Input: part model. Units: mm. Frame: model coordinates. A direction names the side the tool comes from. Round coordinates to 2 decimals unless told otherwise and drop trailing zeros. Write each loop counter-clockwise with the first axis right and the second up, starting at its lowest first coordinate (ties: lowest second). Pieces come first, ordered by that corner, then holes. Notation, with made-up numbers: M -37,-7 L -10,-7 A19 ccw -10,2 Z; hole C 53.5,17.25 d1. An arc over 180 degrees is marked long. Use one line per item in the form item = value. Start each with the question number.
```python
from build123d import *

# Parameters (mm, degrees)
F1_DEPTH  = 3.7
F2_DEPTH  = 55.6
F5_DEPTH  = 5
F7_D      = 3.15
F7_DEPTH  = 10
F7_TIP    = 0.946355475
F9_R      = 3
F10_DEPTH = 10
F12_DEPTH = 5
F11_R     = 2.5
F13_DEPTH = 25
F11_R_2   = 3.5
F14_DEPTH = 1
F15_SIZE  = 4
F16_W     = 4.2
F16_H     = 8
F16_W_2   = 6.1
F16_H_2   = 14
F17_DEPTH = 1
F18_DEPTH = 3
F19_R     = 0.8


with BuildPart() as f1:
    # F0 (on Top) → F1 (new body)
    with BuildSketch(Plane.XY):
        with BuildLine():
            ThreePointArc((43.1, 37.5), (39.2923881554, 46.6923881554), (30.1, 50.5))
            Line((30.1, 50.5), (-35.1, 50.5))
            ThreePointArc((-35.1, 50.5), (-40.7568542495, 48.1568542495), (-43.1, 42.5))
            Line((-43.1, 42.5), (-43.1, -37.5))
            ThreePointArc((-43.1, -37.5), (-39.2923881554, -46.6923881554), (-30.1, -50.5))
            Line((-30.1, -50.5), (30.1, -50.5))
            ThreePointArc((30.1, -50.5), (39.2923881554, -46.6923881554), (43.1, -37.5))
            Line((43.1, -37.5), (43.1, 37.5))
        make_face()
        with BuildLine():
            Line((40.1, 37.5), (40.1, 27.7))
            Line((40.1, 27.7), (40.1, -37.5))
            ThreePointArc((40.1, -37.5), (37.1710678119, -44.5710678119), (30.1, -47.5))
            Line((30.1, -47.5), (-30.1, -47.5))
            ThreePointArc((-30.1, -47.5), (-37.1710678119, -44.5710678119), (-40.1, -37.5))
            Line((-40.1, -37.5), (-40.1, 27.7))
            Line((-40.1, 27.7), (-40.1, 42.5))
            ThreePointArc((-40.1, 42.5), (-38.6355339059, 46.0355339059), (-35.1, 47.5))
            Line((-35.1, 47.5), (30.1, 47.5))
            ThreePointArc((30.1, 47.5), (37.1710678119, 44.5710678119), (40.1, 37.5))
        make_face(mode=Mode.SUBTRACT)
        with BuildLine():
            Line((-30.1, 37.7), (30.1, 37.7))
            ThreePointArc((30.1, 37.7), (37.1710678119, 34.7710678119), (40.1, 27.7))
            Line((40.1, 27.7), (40.1, 37.5))
            ThreePointArc((40.1, 37.5), (37.1710678119, 44.5710678119), (30.1, 47.5))
            Line((30.1, 47.5), (-35.1, 47.5))
            ThreePointArc((-35.1, 47.5), (-38.6355339059, 46.0355339059), (-40.1, 42.5))
            Line((-40.1, 42.5), (-40.1, 27.7))
            ThreePointArc((-40.1, 27.7), (-37.1710678119, 34.7710678119), (-30.1, 37.7))
        make_face()
    extrude(amount=F1_DEPTH)

    # F0 (on Top) → F2 (join)
    with BuildSketch(Plane.XY):
        with BuildLine():
            ThreePointArc((43.1, 37.5), (39.2923881554, 46.6923881554), (30.1, 50.5))
            Line((30.1, 50.5), (-35.1, 50.5))
            ThreePointArc((-35.1, 50.5), (-40.7568542495, 48.1568542495), (-43.1, 42.5))
            Line((-43.1, 42.5), (-43.1, -37.5))
            ThreePointArc((-43.1, -37.5), (-39.2923881554, -46.6923881554), (-30.1, -50.5))
            Line((-30.1, -50.5), (30.1, -50.5))
            ThreePointArc((30.1, -50.5), (39.2923881554, -46.6923881554), (43.1, -37.5))
            Line((43.1, -37.5), (43.1, 37.5))
        make_face()
        with BuildLine():
            Line((40.1, 37.5), (40.1, 27.7))
            Line((40.1, 27.7), (40.1, -37.5))
            ThreePointArc((40.1, -37.5), (37.1710678119, -44.5710678119), (30.1, -47.5))
            Line((30.1, -47.5), (-30.1, -47.5))
            ThreePointArc((-30.1, -47.5), (-37.1710678119, -44.5710678119), (-40.1, -37.5))
            Line((-40.1, -37.5), (-40.1, 27.7))
            Line((-40.1, 27.7), (-40.1, 42.5))
            ThreePointArc((-40.1, 42.5), (-38.6355339059, 46.0355339059), (-35.1, 47.5))
            Line((-35.1, 47.5), (30.1, 47.5))
            ThreePointArc((30.1, 47.5), (37.1710678119, 44.5710678119), (40.1, 37.5))
        make_face(mode=Mode.SUBTRACT)
    extrude(amount=F2_DEPTH)

    # F4 (on offset) → F5 (join, symmetric)
    with BuildSketch(Plane(origin=(0, 0, 0), x_dir=(0, -1, 0), z_dir=(-1, 0, 0))):
        Polygon((47.5, 45.6), (47.5, 55.6), (37.5, 55.6), (37.5, 52.6), align=None)
        Polygon((-37.5, 52.6), (-37.5, 55.6), (-47.5, 55.6), (-47.5, 45.6), align=None)
    extrude(amount=F5_DEPTH, both=True)

    # F7
    with Locations(Plane.XY.offset(55.6)):
        with Locations((0, 42.5), (0, -42.5)):
            Hole(F7_D / 2, depth=F7_DEPTH)
            with Locations((0, 0, -(F7_DEPTH + F7_TIP / 2))):  # 118° drill point
                Cone(0, F7_D / 2, F7_TIP, mode=Mode.SUBTRACT)

    # F9 (on offset) → F10 (cut)
    with BuildSketch(Plane.XY.offset(52.6)):
        with Locations((0, 42.5)):
            Circle(F9_R)
        with Locations((0, -42.5)):
            Circle(F9_R)
    extrude(amount=-F10_DEPTH, mode=Mode.SUBTRACT)

    # F11 (on face) → F12 (join)
    with BuildSketch(Plane.XZ.offset(-47.5)):
        with BuildLine():
            ThreePointArc((-29.1, 37.3270166538), (-26.9377223398, 38.7505102572), (-26.1, 41.2))
            ThreePointArc((-26.1, 41.2), (-32.5494897428, 44.3622776602), (-31.1, 37.3270166538))
            ThreePointArc((-31.1, 37.3270166538), (-30.1, 37.2), (-29.1, 37.3270166538))
        make_face()
        Polygon((-30.1, 44.3754264805), (-27.35, 42.7877132403), (-27.35, 39.6122867597), (-30.1, 38.0245735195), (-32.85, 39.6122867597), (-32.85, 42.7877132403), align=None, mode=Mode.SUBTRACT)
        with BuildLine():
            ThreePointArc((-29.1, 37.3270166538), (-30.1, 37.2), (-31.1, 37.3270166538))
            Line((-31.1, 37.3270166538), (-31.1, 33.2))
            Line((-31.1, 33.2), (-29.1, 33.2))
            Line((-29.1, 33.2), (-29.1, 37.3270166538))
        make_face()
        with BuildLine():
            ThreePointArc((2.9, 37.3270166538), (5.0622776602, 38.7505102572), (5.9, 41.2))
            ThreePointArc((5.9, 41.2), (-0.5494897428, 44.3622776602), (0.9, 37.3270166538))
            ThreePointArc((0.9, 37.3270166538), (1.9, 37.2), (2.9, 37.3270166538))
        make_face()
        Polygon((1.9, 44.3754264805), (4.65, 42.7877132403), (4.65, 39.6122867597), (1.9, 38.0245735195), (-0.85, 39.6122867597), (-0.85, 42.7877132403), align=None, mode=Mode.SUBTRACT)
        with BuildLine():
            ThreePointArc((2.9, 37.3270166538), (1.9, 37.2), (0.9, 37.3270166538))
            Line((0.9, 37.3270166538), (0.9, 33.2))
            Line((0.9, 33.2), (2.9, 33.2))
            Line((2.9, 33.2), (2.9, 37.3270166538))
        make_face()
        with BuildLine():
            ThreePointArc((-27.1, 8.3270166538), (-24.9377223398, 9.7505102572), (-24.1, 12.2))
            ThreePointArc((-24.1, 12.2), (-30.5494897428, 15.3622776602), (-29.1, 8.3270166538))
            ThreePointArc((-29.1, 8.3270166538), (-28.1, 8.2), (-27.1, 8.3270166538))
        make_face()
        Polygon((-28.1, 15.3754264805), (-25.35, 13.7877132403), (-25.35, 10.6122867597), (-28.1, 9.0245735195), (-30.85, 10.6122867597), (-30.85, 13.7877132403), align=None, mode=Mode.SUBTRACT)
        with BuildLine():
            ThreePointArc((-27.1, 8.3270166538), (-28.1, 8.2), (-29.1, 8.3270166538))
            Line((-29.1, 8.3270166538), (-29.1, 6.2))
            Line((-29.1, 6.2), (-27.1, 6.2))
            Line((-27.1, 6.2), (-27.1, 8.3270166538))
        make_face()
        with BuildLine():
            ThreePointArc((5.9, 8.3270166538), (8.0622776602, 9.7505102572), (8.9, 12.2))
            ThreePointArc((8.9, 12.2), (2.4505102572, 15.3622776602), (3.9, 8.3270166538))
            ThreePointArc((3.9, 8.3270166538), (4.9, 8.2), (5.9, 8.3270166538))
        make_face()
        Polygon((4.9, 15.3754264805), (7.65, 13.7877132403), (7.65, 10.6122867597), (4.9, 9.0245735195), (2.15, 10.6122867597), (2.15, 13.7877132403), align=None, mode=Mode.SUBTRACT)
        with BuildLine():
            ThreePointArc((5.9, 8.3270166538), (4.9, 8.2), (3.9, 8.3270166538))
            Line((3.9, 8.3270166538), (3.9, 6.2))
            Line((3.9, 6.2), (5.9, 6.2))
            Line((5.9, 6.2), (5.9, 8.3270166538))
        make_face()
    extrude(amount=F12_DEPTH)

    # F11 (on face) → F13 (cut)
    with BuildSketch(Plane.XZ.offset(-47.5)):
        with Locations((-18.1, 16.7)):
            Circle(F11_R)
    extrude(amount=-F13_DEPTH, mode=Mode.SUBTRACT)

    # F11 (on face) → F14 (cut)
    with BuildSketch(Plane.XZ.offset(-47.5)):
        with Locations((-18.1, 16.7)):
            Circle(F11_R_2)
        with Locations((-18.1, 16.7)):
            Circle(F11_R, mode=Mode.SUBTRACT)
        with Locations((-18.1, 16.7)):
            Circle(F11_R)
    extrude(amount=-F14_DEPTH, mode=Mode.SUBTRACT)

    # F15
    f15_edges = [f1.edges().sort_by_distance(p)[0] for p in [
        (1.9, 42.5, 33.2),
        (-30.1, 42.5, 33.2),
    ]]
    chamfer(f15_edges, length=F15_SIZE)

    # F16 (on face) → F17 (cut)
    with BuildSketch(Plane.YZ.offset(-40.1)):
        Polygon((27.7, 3.7), (42.5, 3.7), (42.5, 48.7), (27.5, 48.7), (27.5, 3.7), align=None)
        with Locations((39.5, 14)):
            Rectangle(F16_W, F16_H, mode=Mode.SUBTRACT)
        with Locations((38.55, 32.2)):
            Rectangle(F16_W_2, F16_H_2, mode=Mode.SUBTRACT)
    extrude(amount=-F17_DEPTH, mode=Mode.SUBTRACT)

    # F16 (on face) → F18 (cut)
    with BuildSketch(Plane.YZ.offset(-40.1)):
        with Locations((38.55, 32.2)):
            Rectangle(F16_W_2, F16_H_2)
        with Locations((39.5, 14)):
            Rectangle(F16_W, F16_H)
    extrude(amount=-F18_DEPTH, mode=Mode.SUBTRACT)

    # F19
    f19_edges = [f1.edges().sort_by_distance(p)[0] for p in [
        (-42.1, 37.4, 18),
        (-42.1, 37.4, 10),
    ]]
    fillet(f19_edges, radius=F19_R)


solid = f1.part
```
Item 1: First-contact query: pin 1 (2.5 mm diameter, centred on y = 45, z = 12, fed in from -X); pin 2 (1.7 mm diameter, centred on y = 44, z = 7.5, fed in from +X); pin 3 (1.6 mm diameter, centred on x = -28.5, y = 44.5, fed in from -Z); pin 4 (1.2 mm diameter, centred on y = 45.5, z = 34.5, fed in from +X). Flat tips, straight axial feed; report the tip coordinate or a pass-through.
Item 2: Ray query, line 1 (Y direction, x = 0, z = 54.6) (3 decimals); line 2 (X direction, y = 18, z = 49); line 3 (Y direction, x = -13.5, z = 31). Return the intervals inside material, ascending. Write a range as from..to.
Item 3: Cut plane D-D (x = 33). Output: boundary loops of the cut face in (y, z).
Item 4: Cut plane C-C (z = 28.5). Output: boundary loops of the cut face in (x, y).
Item 5: Cut plane B-B (y = 30). Output: boundary loops of the cut face in (x, z).
Item 6: Cut plane A-A (x = -9.5). Output: boundary loops of the cut face in (y, z).
Item 7: Draft query along Y for faces 1 (the face through (39.191, -46.793, 27.411)), 2 (the face through (5, 47.5, 12)), 3 (the face through (0, 41, 0)), 4 (the face through (40.1, 1, 27)). Return one class per face: +Y half, -Y half, draft (parallel to the pull), parting line (faces both ways), or undercut.
Item 8: Reachability of faces 5 (the face through (-0.391, 45.474, 50.442)), 6 (the face through (0, -37.5, 54)), 7 (the face through (-39.393, -46.591, 27.411)), 8 (the face through (-5, 44, 52)) from +Z, -Z, +X, -X, +Y, -Y: full face, straight path, thin tool, end or side. Return the list, or none.
Final values:
q1.pin_1 = -43
q1.pin_2 = 41.81
q1.pin_3 = 0
q1.pin_4 = 40.79
q2.line_1 = -50.5..-44.075, -40.925..-37.5, 37.5..40.925, 44.075..50.5
q2.line_2 = -43.1..-40.1, 40.1..43.1
q2.line_3 = -50.5..-47.5, 47.5..50.5
q3.outline = M -50.17,0 L -47.07,0 L -47.07,55.6 L -50.17,55.6 Z; M 37.27,0 L 50.17,0 L 50.17,55.6 L 47.07,55.6 L 47.07,3.7 L 37.27,3.7 Z
q4.outline = M -43.1,-37.5 A13 ccw -30.1,-50.5 L 30.1,-50.5 A13 ccw 43.1,-37.5 L 43.1,37.5 A13 ccw 30.1,50.5 L -35.1,50.5 A8 ccw -43.1,42.5 L -43.1,41.6 L -41.1,41.6 L -41.1,42.5 L -40.1,42.5 A5 cw -35.1,47.5 L 30.1,47.5 A10 cw 40.1,37.5 L 40.1,-37.5 A10 cw 30.1,-47.5 L -30.1,-47.5 A10 cw -40.1,-37.5 L -40.1,27.5 L -41.1,27.5 L -41.1,35.5 L -43.1,35.5 Z
q5.outline = M -43.1,0 L -39.83,0 L -39.83,3.7 L -41.1,3.7 L -41.1,48.7 L -40.1,48.7 L -40.1,55.6 L -43.1,55.6 Z; M 39.83,0 L 43.1,0 L 43.1,55.6 L 40.1,55.6 L 40.1,3.7 L 39.83,3.7 Z
q6.outline = M -50.5,0 L -47.5,0 L -47.5,55.6 L -50.5,55.6 Z; M 37.7,0 L 50.5,0 L 50.5,55.6 L 47.5,55.6 L 47.5,3.7 L 37.7,3.7 Z
q7.face_1 = -Y half
q7.face_2 = undercut
q7.face_3 = draft
q7.face_4 = undercut
q8.face_5 = none
q8.face_6 = +Z, -Z
q8.face_7 = +Z, -Z, -X, -Y
q8.face_8 = +Z
